For this review, take the finished solid that the model builds, in its own axes (mm). A direction names the side the tool comes from. Give positions to 0.01 mm unless a question says otherwise; leave off trailing zeros. Write each loop counter-clockwise with the first axis right and the second up, starting at its lowest first coordinate (ties: lowest second). Pieces come first, ordered by that corner, then holes. Notation, with made-up numbers: (30, 68.25) -> (53, 68.25) arc R36 ccw to (53, 106.25) -> close; hole circle Ø9 at (0.5, -40). An arc over 180 degrees is marked (long way). Return JSON: item names as keys, results as strings.
from build123d import *

# Parameters (mm, degrees)
SKETCH1_R           = 5.5
BOSS_EXTRUDE1_DEPTH = 12
SKETCH2_W           = 3
SKETCH2_H           = 2.6
BOSS_EXTRUDE2_DEPTH = 12
CUT_EXTRUDE1_DEPTH  = 3.8
SKETCH5_R           = 2.75
CUT_EXTRUDE3_DEPTH  = 17.65


with BuildPart() as part:
    # Sketch1 → Boss-Extrude1 (new body)
    with BuildSketch(Plane(origin=(0, 0, 0), x_dir=(1, 0, 0), z_dir=(0, 1, 0))):
        Circle(SKETCH1_R)
    extrude(amount=BOSS_EXTRUDE1_DEPTH)

    # Sketch2 → Boss-Extrude2 (add)
    with BuildSketch(Plane(origin=(0, 12, 0), x_dir=(1, 0, 0), z_dir=(0, 1, 0))):
        with Locations((4.8, -0.147270773)):
            Rectangle(SKETCH2_W, SKETCH2_H)
    extrude(amount=-BOSS_EXTRUDE2_DEPTH)

    # Sketch3 → Cut-Extrude1 (cut)
    with BuildSketch(Plane(origin=(0, 0, 0), x_dir=(-1, 0, 0), z_dir=(0, -1, 0))):
        Polygon((-1.891599986, 4.086789631), (-4.485063634, 0.405221174), (-2.593463648, -3.681568458), (1.891599986, -4.086789631), (4.485063634, -0.405221174), (2.593463648, 3.681568458), align=None)
    extrude(amount=-CUT_EXTRUDE1_DEPTH, mode=Mode.SUBTRACT)

    # Sketch5 → Cut-Extrude3 (cut)
    with BuildSketch(Plane(origin=(0, 12, 0), x_dir=(1, 0, 0), z_dir=(0, 1, 0))):
        Circle(SKETCH5_R)
    extrude(amount=-CUT_EXTRUDE3_DEPTH, mode=Mode.SUBTRACT)


solid = part.part
1. For pin 1 (1 mm diameter, centred on x = 2.5, y = 4, fed in from +Z); pin 2 (0.8 mm diameter, centred on x = 6, y = 7, fed in from +Z); pin 3 (2 mm diameter, centred on x = 2.5, y = 9, fed in from -Z), all flat-tipped, find the tip position at first contact; note any pin that passes through.
Results found:
{"pin 1": "stops at z = 5.12", "pin 2": "stops at z = 1.45", "pin 3": "stops at z = -5.29"}
2. To check wall thickness, follow probe 1 along X at (y, z) = (8.25, 0); probe 2 along Z at (x, y) = (0, 9.25); probe 3 along Y at (x, z) = (-2, -2.75). State the ranges of each line that lie inside material, in increasing order.
Results found:
{"probe 1": "x = -5.5 to -2.75, 2.75 to 6.3", "probe 2": "z = -5.5 to -2.75, 2.75 to 5.5", "probe 3": "y = 3.8 to 12"}
3. Add section D-D, the plane z = -3. State the section outline as (x, y) points, plus the area to 3 significant figures.
Results found:
{"outline": "(-4.61, 0) -> (-2.91, 0) -> (-2.91, 3.8) -> (2.66, 3.8) -> (2.66, 0) -> (4.61, 0) -> (4.61, 12) -> (-4.61, 12) -> close", "area": "89.5 mm²"}
4. For faces 4 (the flat face through (4, 0, -2)), 5 (the flat face through (3.553, 1.873, 1.61)), 6 (the flat face through (6, 6, -1.153)), list the 3-axis set-ups (+Z, -Z, +X, -X, +Y, -Y) from which the entire face can be reached by the end or side of a thin tool; tool diameter is ignored.
Results found:
{"face 4": "+Z, -Z, +X, -X, -Y", "face 5": "-Y", "face 6": "-Z, +X, +Y, -Y"}
5. Add section A-A, the plane x = -0.5. State the section outline as (y, z) points.
Results found:
{"outline": "(0, -5.48) -> (12, -5.48) -> (12, -2.7) -> (3.8, -2.7) -> (3.8, -3.87) -> (0, -3.87) -> close; (0, 3.96) -> (3.8, 3.96) -> (3.8, 2.7) -> (12, 2.7) -> (12, 5.48) -> (0, 5.48) -> close"}
6. The part is to be moulded in two halves that separate along X. For faces 1 (the flat face through (6.3, 6, 0)), 2 (the cylindrical face through (-0.596, 7.957, 2.685)), 3 (the flat face through (6, 6, 1.447)), say which applies: +X half, -X half, draft (parallel to the pull), parting line (faces both ways), or undercut.
Results found:
{"face 1": "+X half", "face 2": "undercut", "face 3": "draft"}
7. Add section B-B, the plane y = 2.25. State the section outline as (x, z) points.
Results found:
{"outline": "(5.31, 1.45) arc R5.5 ccw (long way) to (5.38, -1.15) -> (6.3, -1.15) -> (6.3, 1.45) -> close; hole (-4.49, 0.41) -> (-2.59, -3.68) -> (1.89, -4.09) -> (4.49, -0.41) -> (2.59, 3.68) -> (-1.89, 4.09) -> close"}
8. Add section C-C, the plane z = 0. State the section outline as (x, y) points, plus the area to 3 significant figures.
Results found:
{"outline": "(-5.5, 0) -> (-4.3, 0) -> (-4.3, 3.8) -> (-2.75, 3.8) -> (-2.75, 12) -> (-5.5, 12) -> close; (2.75, 3.8) -> (4.3, 3.8) -> (4.3, 0) -> (6.3, 0) -> (6.3, 12) -> (2.75, 12) -> close", "area": "63.8 mm²"}
